Verification items for the finished model (mm, model axes). A direction names the side the tool comes from. Coordinates: 2 decimals unless noted, no trailing zeros. Order: outer loops, then holes, each group sorted by start corner. A loop starts at its lowest first (then second) coordinate and runs counter-clockwise, first axis right, second up. Notation, with made-up numbers: M 13.5,16 L 26.5,16 A21 cw 26.5,53 Z; hole C 19,79.5 d10. An arc over 180 degrees is marked long. Return JSON: item names as keys, results as strings.
```python
from build123d import *

# Parameters (mm, degrees)
PAD_DEPTH       = 20
SKETCH001_W     = 75
SKETCH001_H     = 75
PAD001_DEPTH    = 3
SKETCH003_W     = 10
SKETCH003_H     = 4.5
POCKET001_DEPTH = 3.535534
SKETCH004_W     = 3
SKETCH004_H     = 8
PAD002_DEPTH    = 7
PAD003_DEPTH    = 5
SKETCH006_W     = 12
SKETCH006_H     = 8
POCKET002_DEPTH = 3.535534
SKETCH002_R     = 3.5
POCKET_DEPTH    = 8


with BuildPart() as part:
    # Sketch → Pad (new body)
    with BuildSketch(Plane.XY):
        with BuildLine():
            Line((-35, 40), (35, 40))
            ThreePointArc((40, 35), (38.535534, 38.535534), (35, 40))
            Line((40, 35), (40, -35))
            ThreePointArc((35, -40), (38.535534, -38.535534), (40, -35))
            Line((35, -40), (-35, -40))
            ThreePointArc((-40, -35), (-38.535534, -38.535534), (-35, -40))
            Line((-40, -35), (-40, 35))
            ThreePointArc((-35, 40), (-38.535534, 38.535534), (-40, 35))
        make_face()
        with BuildLine():
            Line((-31.464466, 36.464466), (31.464466, 36.464466))
            ThreePointArc((36.464466, 31.464466), (35, 35), (31.464466, 36.464466))
            Line((36.464466, 31.464466), (36.464466, -31.464466))
            ThreePointArc((31.464466, -36.464466), (35, -35), (36.464466, -31.464466))
            Line((31.464466, -36.464466), (-31.464466, -36.464466))
            ThreePointArc((-36.464466, -31.464466), (-35, -35), (-31.464466, -36.464466))
            Line((-36.464466, -31.464466), (-36.464466, 31.464466))
            ThreePointArc((-31.464466, 36.464466), (-35, 35), (-36.464466, 31.464466))
        make_face(mode=Mode.SUBTRACT)
    extrude(amount=PAD_DEPTH)

    # Sketch001 (on Face17 of Pad) → Pad001 (join)
    with BuildSketch(Plane(origin=(0, 0, 0), x_dir=(1, 0, 0), z_dir=(0, 0, -1))):
        Rectangle(SKETCH001_W, SKETCH001_H)
    extrude(amount=-PAD001_DEPTH)

    # Sketch003 → Pocket001 (cut)
    with BuildSketch(Plane(origin=(0, -36.464466, 0), x_dir=(-1, 0, 0), z_dir=(0, 1, 0))):
        with Locations((-16.464466, 5.75)):
            Rectangle(SKETCH003_W, SKETCH003_H)
    extrude(amount=-POCKET001_DEPTH, mode=Mode.SUBTRACT)

    # Sketch004 (on Face15 of Pocket001) → Pad002 (join)
    with BuildSketch(Plane(origin=(0, -36.464466, 0), x_dir=(-1, 0, 0), z_dir=(0, 1, 0))):
        with Locations((-24.464466, 7)):
            Rectangle(SKETCH004_W, SKETCH004_H)
        with Locations((-8.464466, 7)):
            Rectangle(SKETCH004_W, SKETCH004_H)
    extrude(amount=PAD002_DEPTH)

    # Sketch005 (on Face25 of Pad002) → Pad003 (join)
    with BuildSketch(Plane.XY.offset(3)):
        with BuildLine():
            ThreePointArc((-8.660254, 5), (0, -10), (8.660254, 5))
            Line((-8.660254, 5), (8.660254, 5))
        make_face()
    extrude(amount=PAD003_DEPTH)

    # Sketch006 → Pocket002 (cut)
    with BuildSketch(Plane.YZ.offset(-36.464466)):
        with Locations((20.464466, 7.1)):
            Rectangle(SKETCH006_W, SKETCH006_H)
    extrude(amount=-POCKET002_DEPTH, mode=Mode.SUBTRACT)

    # Sketch002 (on Face20 of Pad001) → Pocket (cut)
    with BuildSketch(Plane(origin=(0, 0, 0), x_dir=(1, 0, 0), z_dir=(0, 0, -1))):
        with Locations((31.464466, 31.464466)):
            Circle(SKETCH002_R)
        with BuildLine():
            ThreePointArc((-3.307189, 3.75), (0, -5), (3.307189, 3.75))
            Line((-3.307189, 3.75), (3.307189, 3.75))
        make_face()
    extrude(amount=-POCKET_DEPTH, mode=Mode.SUBTRACT)


solid = part.part
```
Q1. Draft check along X on faces 4 (the face through (0, -38, 20)), 5 (the face through (-39, -38, 10)), 6 (the face through (0, -3.75, 4)). Enter one of: pulls with the +X half, pulls with the -X half, needs draft (parallel to the pull), parting line crosses it, or undercut.
Values:
{"face 4": "needs draft", "face 5": "pulls with the -X half", "face 6": "undercut"}
Q2. Cross-section at B-B, the plane x = -18. Record the boundary of the cut face in (y, z), and give its area (3 significant figures).
Values:
{"outline": "M -40,0 L 40,0 L 40,20 L 36.46,20 L 36.46,3 L -36.46,3 L -36.46,20 L -40,20 Z", "area": "360 mm^2"}
Q3. Cross-section at D-D, the plane x = 29.5. Record the boundary of the cut face in (y, z).
Values:
{"outline": "M -40,0 L -34.36,0 L -34.36,3 L -36.46,3 L -36.46,20 L -40,20 Z; M -28.57,0 L 40,0 L 40,20 L 36.46,20 L 36.46,3 L -28.57,3 Z"}
Q4. Go/stop test with flat-tipped pins: pin 1 (8 mm diameter, centred on x = -1.5, y = -4.5, fed in from +Z); pin 2 (4 mm diameter, centred on x = -0.5, y = 30.5, fed in from +Z); pin 3 (0.9 mm diameter, centred on x = 25, y = -33.5, fed in from +Z). Record where each tip stops, or that it passes through.
Values:
{"pin 1": "z = 8", "pin 2": "z = 3", "pin 3": "z = 11"}
Q5. Material ranges on line 1 along X through (y, z) = (0, 5); line 2 along Y through (x, z) = (-12, 6), recorded low to high.
Values:
{"line 1": "-40 to -36.46, -10 to -5, 5 to 10, 36.46 to 40", "line 2": "-40 to -36.46, 36.46 to 40"}
Q6. Cross-section at A-A, the plane y = 0. Record the boundary of the cut face in (x, z).
Values:
{"outline": "M -40,0 L -5,0 L -5,8 L -10,8 L -10,3 L -36.46,3 L -36.46,20 L -40,20 Z; M 5,0 L 40,0 L 40,20 L 36.46,20 L 36.46,3 L 10,3 L 10,8 L 5,8 Z"}
Q7. Tool access check on faces 1 (the face through (0, -36.464, 11)), 2 (the face through (11.464, -38, 6)), 3 (the face through (-38, 20, 3.1)). Record the directions out of +Z, -Z, +X, -X, +Y, -Y that give a thin tool (end or side, any length) a straight path to the whole face; none if there is none.
Values:
{"face 1": "+Z", "face 2": "-Y", "face 3": "-X"}
